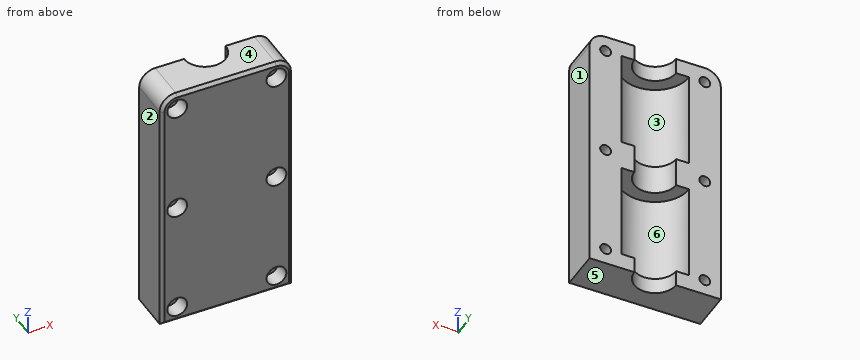
```python
from build123d import *

# Parameters (mm, degrees)
PAD_DEPTH       = 40
SKETCH001_R     = 1.7
POCKET_DEPTH    = 13.501
SKETCH002_R     = 10.6
POCKET001_DEPTH = 30.4
SKETCH003_R     = 10.6
POCKET002_DEPTH = 30.4
FILLET_R        = 5
CHAMFER_SIZE    = 1
SKETCH004_R     = 3.1
POCKET003_DEPTH = 5


with BuildPart() as part:
    # Sketch → Pad (new body, symmetric)
    with BuildSketch(Plane.XY):
        with BuildLine():
            Line((-20.5, -13.5), (20.5, -13.5))
            Line((20.5, -13.5), (20.5, 0))
            Line((20.5, 0), (6.5, 0))
            ThreePointArc((-6.5, 0), (0, -6.5), (6.5, 0))
            Line((-6.5, 0), (-20.5, 0))
            Line((-20.5, 0), (-20.5, -13.5))
        make_face()
    extrude(amount=PAD_DEPTH, both=True)

    # Sketch001 → Pocket (cut, through all)
    with BuildSketch(Plane.XZ):
        with Locations((-15.5, 35)):
            Circle(SKETCH001_R)
        with Locations((-15.5, 0)):
            Circle(SKETCH001_R)
        with Locations((-15.5, -35)):
            Circle(SKETCH001_R)
        with Locations((15.5, -35)):
            Circle(SKETCH001_R)
        with Locations((15.5, 0)):
            Circle(SKETCH001_R)
        with Locations((15.5, 35)):
            Circle(SKETCH001_R)
    extrude(amount=POCKET_DEPTH, mode=Mode.SUBTRACT)

    # Sketch002 (on DatumPlane) → Pocket001 (cut)
    with BuildSketch(Plane.XY.offset(35)):
        Circle(SKETCH002_R)
    extrude(amount=-POCKET001_DEPTH, mode=Mode.SUBTRACT)

    # Sketch003 (on DatumPlane) → Pocket002 (cut)
    with BuildSketch(Plane.XY.offset(-35)):
        Circle(SKETCH003_R)
    extrude(amount=POCKET002_DEPTH, mode=Mode.SUBTRACT)

    # Fillet
    fillet_edges = [part.edges().sort_by_distance(p)[0] for p in [
        (-20.5, -6.75, 40),
        (20.5, -6.75, 40),
    ]]
    fillet(fillet_edges, radius=FILLET_R)

    # Chamfer
    chamfer_edges = [part.edges().sort_by_distance(p)[0] for p in [
        (-20.5, -13.5, -2.5),
        (0, -13.5, -40),
    ]]
    chamfer(chamfer_edges, length=CHAMFER_SIZE)

    # Sketch004 (on Face1 of Chamfer) → Pocket003 (cut)
    with BuildSketch(Plane.XZ.offset(13.5)):
        with Locations((-15.5, 35)):
            Circle(SKETCH004_R)
        with Locations((15.5, 35)):
            Circle(SKETCH004_R)
        with Locations((-15.5, -35)):
            Circle(SKETCH004_R)
        with Locations((-15.5, 0)):
            Circle(SKETCH004_R)
        with Locations((15.5, 0)):
            Circle(SKETCH004_R)
        with Locations((15.5, -35)):
            Circle(SKETCH004_R)
    extrude(amount=-POCKET003_DEPTH, mode=Mode.SUBTRACT)


solid = part.part
```
Here's how the part is built. I have some questions about the finished solid (model axes, mm). Face numbers are marked on the shaded views. A direction names the side the tool comes from. Round coordinates to 2 decimals unless told otherwise and drop trailing zeros. Loops run counter-clockwise (first coordinate to the right, second up) from the corner with the lowest first, then second, coordinate; pieces in that order, holes last.
1. For the marked faces 5 and 6, which set-ups out of +Z, -Z, +X, -X, +Y, -Y let a thin tool reach every point of the face, with its end or its side?
Answers:
face 5: -Z, +X, -X, +Y, -Y
face 6: +Y
2. Suppose I cut it at A-A, the plane z = 0. Please give me the cut outline in (x, y), and give its area (3 significant figures).
Answers:
outline: (-20.5, -12.5) - (-19.5, -13.5) - (-18.6, -13.5) - (-18.6, -8.5) - (-17.2, -8.5) - (-17.2, 0) - (-20.5, 0) - close; (-13.8, -8.5) - (-12.4, -8.5) - (-12.4, -13.5) - (12.4, -13.5) - (12.4, -8.5) - (13.8, -8.5) - (13.8, 0) - (6.5, 0) arc R6.5 cw to (-6.5, 0) - (-13.8, 0) - close; (17.2, -8.5) - (18.6, -8.5) - (18.6, -13.5) - (19.5, -13.5) - (20.5, -12.5) - (20.5, 0) - (17.2, 0) - close
area: 366 mm2
3. Suppose I cut it at B-B, the plane x = 1.5. Please give me the cut outline in (y, z), and give its area (3 significant figures).
Answers:
outline: (-13.5, -39) - (-12.5, -40) - (-6.32, -40) - (-6.32, -35) - (-10.49, -35) - (-10.49, -4.6) - (-6.32, -4.6) - (-6.32, 4.6) - (-10.49, 4.6) - (-10.49, 35) - (-6.32, 35) - (-6.32, 40) - (-12.5, 40) - (-13.5, 39) - close
area: 320 mm2
4. Suppose I cut it at D-D, the plane x = -4. Please give me the cut outline in (y, z), and give its area (3 significant figures).
Answers:
outline: (-13.5, -39) - (-12.5, -40) - (-5.12, -40) - (-5.12, -35) - (-9.82, -35) - (-9.82, -4.6) - (-5.12, -4.6) - (-5.12, 4.6) - (-9.82, 4.6) - (-9.82, 35) - (-5.12, 35) - (-5.12, 40) - (-12.5, 40) - (-13.5, 39) - close
area: 384 mm2
5. Thinking about a two-plate mould opening in X: for the marked faces 1, 2, 3 and 4, which applies, released by +X, released by -X, zero draft, split by the parting line, or undercut?
Answers:
face 1: released by +X
face 2: released by -X
face 3: undercut
face 4: zero draft
6. Suppose I cut it at C-C, the plane z = -8.5. Please give me the cut outline in (x, y).
Answers:
outline: (-20.5, -12.5) - (-19.5, -13.5) - (19.5, -13.5) - (20.5, -12.5) - (20.5, 0) - (10.6, 0) arc R10.6 cw to (-10.6, 0) - (-20.5, 0) - close
7. If I drill on probe 1 along Z at (x, y) = (7, -5); probe 2 along Z at (x, y) = (15.5, -1.75); probe 3 along Z at (x, y) = (15.5, -11.2), over which ranges is the centre line in solid material (lowest first)?
Answers:
probe 1: z = -40 to -35, -4.6 to 4.6, 35 to 40
probe 2: z = -40 to -36.7, -33.3 to -1.7, 1.7 to 33.3, 36.7 to 40
probe 3: z = -40 to -38.1, -31.9 to -3.1, 3.1 to 31.9, 38.1 to 40
8. Will this pin go through, and if not, where does the flat tip stop? pin 1 (1.9 mm diameter, centred on x = -14.5, z = -35, fed in from -Y).
Answers:
pin 1: stops at y = -8.5
